Design review of the part built by this model. Coordinates are the model's own, in mm. A direction names the side the tool comes from. Coordinates: 2 decimals unless noted, no trailing zeros. Loops run counter-clockwise (first coordinate to the right, second up) from the corner with the lowest first, then second, coordinate; pieces in that order, holes last. Notation, with made-up numbers: (-25.5, 20) -> (-18.5, 20) arc R23 cw to (-18.5, 54) -> close; hole circle Ø9 at (15.5, -4.75). An arc over 180 degrees is marked (long way). One line per item, written item: value. Start each with the question number.
1. Insertion check: pin 1 (6 mm diameter, centred on x = 3.5, y = -13, fed in from +Z); pin 2 (1.6 mm diameter, centred on x = 1.5, z = 4.5, fed in from -Y); pin 3 (1 mm diameter, centred on x = -2.5, z = -4.5, fed in from -Y). Each pin has a flat end and moves straight along its axis. Give the tip position at first contact, or say it passes through.
2. For probe 1 along Y at (x, z) = (-4.75, -1.75); probe 2 along Z at (x, y) = (-2, -54); probe 3 along Y at (x, z) = (-3.5, 0.75), list the stretches that pass through material, from the lowest coordinate up.
3. Machinability: for faces 1 (the flat face through (0, -60.3, 0)), 2 (the flat face through (3, -5.3, -3)), which of the approach directions +Z, -Z, +X, -X, +Y, -Y give a long, thin tool a straight path to every point of the face, cutting with its end or side? Answer none if there is none.
4. Add section A-A on y = -26. Write out the cut boundary in (x, z), plus the area to 3 significant figures.
```python
from build123d import *

# Parameters (mm, degrees)
BOSS_EXTRUDE1_DEPTH = 5.3
SKETCH2_OUTSIDE_W   = 21.122
SKETCH2_OUTSIDE_H   = 19.11
SKETCH2_OUTSIDE_R   = 6.5
CUT_EXTRUDE1_DEPTH  = 0.265
SKETCH3_R           = 4
BOSS_EXTRUDE2_DEPTH = 55
CHAMFER1_SIZE       = 0.8


with BuildPart() as part:
    # Sketch1 → Boss-Extrude1 (new body)
    with BuildSketch(Plane(origin=(0, 0, 0), x_dir=(1, 0, 0), z_dir=(0, 1, 0))):
        Polygon((7.505553499, 0), (3.75277675, 6.5), (-3.75277675, 6.5), (-7.505553499, 0), (-3.75277675, -6.5), (3.75277675, -6.5), align=None)
    extrude(amount=-BOSS_EXTRUDE1_DEPTH)

    # Sketch4 → Cut-Revolve1 (revolve, cut)
    with BuildSketch(Plane(origin=(0, 0, 0), x_dir=(0, 0, -1), z_dir=(1, 0, 0))):
        Polygon((-6.5, 0), (-8.15, 0), (-8.15, -1.65), align=None)
        Polygon((-8.15, -3.65), (-6.5, -5.3), (-8.15, -5.3), align=None)
    revolve(axis=Axis((0, 0, 0), (0, -1, 0)), mode=Mode.SUBTRACT)

    # Sketch2 outside → Cut-Extrude1 (cut)
    with BuildSketch(Plane.XZ.offset(5.3)):
        Rectangle(SKETCH2_OUTSIDE_W, SKETCH2_OUTSIDE_H)
        with Locations(Location((0, 0, 0), (0, 0, 90))):
            Circle(SKETCH2_OUTSIDE_R, mode=Mode.SUBTRACT)
    extrude(amount=-CUT_EXTRUDE1_DEPTH, mode=Mode.SUBTRACT)

    # Sketch3 → Boss-Extrude2 (add)
    with BuildSketch(Plane.XZ.offset(5.3)):
        with Locations(Location((0, 0, 0), (0, 0, 90))):
            Circle(SKETCH3_R)
    extrude(amount=BOSS_EXTRUDE2_DEPTH)

    # Chamfer1
    chamfer1_edges = [part.edges().sort_by_distance(p)[0] for p in [
        (0, -60.3, -4),
    ]]
    chamfer(chamfer1_edges, length=CHAMFER1_SIZE)


solid = part.part
```
Worked answers:
1. pin 1: stops at z = 3.97
1. pin 2: stops at y = -59.56
1. pin 3: stops at y = -5.3
2. probe 1: y = -5.3 to 0
2. probe 2: z = -3.46 to 3.46
2. probe 3: y = -59.92 to 0
3. face 1: +Z, -Z, +X, -X, -Y
3. face 2: -Y
4. outline: circle Ø8 at (0, 0)
4. area: 50.3 mm²
